Input: part model. Units: mm. Frame: model coordinates. A direction names the side the tool comes from. Coordinates: 2 decimals unless noted, no trailing zeros. Loops run counter-clockwise (first coordinate to the right, second up) from the corner with the lowest first, then second, coordinate; pieces in that order, holes last. Notation, with made-up numbers: (31.25, -26) - (68.25, -26) arc R21 ccw to (68.25, -2) - close; hole circle Ø2 at (72, 69). An arc over 180 degrees is marked (long way). Use a Markdown table: item, result. Add a question column.
1. Section query C-C on x = -8.75. Return the cut outline in (y, z).
2. Access query for faces 1 (the face through (-13.3, -6, 0)), 2 (the face through (-4.01, -5.69, 39.33)), 3 (the face through (-8.3, -6, -1)), 4 (the face through (-5, -6, 25)). Directions: +Z, -Z, +X, -X, +Y, -Y. A direction counts if a zero-diameter tool reaches every point of the face in a straight line with its end or side. Return the directions, or none.
3. Section query B-B on y = -6. Return the cut outline in (x, z), then the cut area to 3 significant figures.
4. Contact query for flat-ended pins moving along their axis: P1, Ø1.4, axis at y = -7, z = 37, coming from the -X side; P2, Ø4, axis at x = -11, y = -8.5, coming from the +Z side; P3, Ø6.5, axis at x = -2.5, y = -4, coming from the -Z side. Output: stop coordinate, or through.
5. Draft query along Z for faces 5 (the face through (-10.84, -6.62, -2.5)), 6 (the face through (-4, -5.2, 37)), 7 (the face through (-9, -6, 5)), 8 (the face through (-4, -6, 0)). Return one class per face: released by +Z, released by -Z, zero draft, split by the parting line, or undercut.
6. Ray query, L1, parallel to Z at x = -3.5, y = -6; L2, parallel to X at y = -3.75, z = 29; L3, parallel to Z at x = -2.25, y = -1.25. Return the intervals inside material, ascending. Write a range as [from, to].
7. Section query A-A on z = -2.7. Return the cut outline in (x, y).
8. Section query D-D on y = -1.75. Return the cut outline in (x, z).
```python
from build123d import *

# Parameters (mm, degrees)
F1_DEPTH = 12
F2_R     = 0.65
F3_DEPTH = 5
F4_R     = 2.35
F4_R_2   = 0.8
F5_DEPTH = 2


with BuildPart() as f1:
    # F0 (on Front) → F1 (new body)
    with BuildSketch(Plane.XZ):
        Polygon((-13.3, 5), (-13.3, -5), (-8.3, -5), (-8.3, 0), (0, 0), (0, 45), (-5, 45), (-5, 5), align=None)
    extrude(amount=F1_DEPTH)

    # F2 (on face) → F3 (cut)
    with BuildSketch(Plane(origin=(-13.3, 0, 0), x_dir=(0, -1, 0), z_dir=(-1, 0, 0))):
        with Locations((6, -2.7)):
            Circle(F2_R)
    extrude(amount=-F3_DEPTH, mode=Mode.SUBTRACT)

    # F4 (on face) → F5 (cut)
    with BuildSketch(Plane(origin=(-5, 0, 0), x_dir=(0, -1, 0), z_dir=(-1, 0, 0))):
        with Locations((6, 37)):
            Circle(F4_R)
        with Locations((6, 37)):
            Circle(F4_R_2, mode=Mode.SUBTRACT)
    extrude(amount=-F5_DEPTH, mode=Mode.SUBTRACT)


solid = f1.part
```
Resolved:
| question | item | result |
|---|---|---|
| 1 | outline | (-12, -5) - (0, -5) - (0, 5) - (-12, 5) - close; hole circle Ø1.3 at (-6, -2.7) |
| 2 | face 1 | +Z, -Z, -X, +Y, -Y |
| 2 | face 2 | -X |
| 2 | face 3 | -Z, +X, +Y, -Y |
| 2 | face 4 | +Z, -X, +Y, -Y |
| 3 | outline | (-13.3, -5) - (-8.3, -5) - (-8.3, -3.35) - (-13.3, -3.35) - close; (-13.3, -2.05) - (-8.3, -2.05) - (-8.3, 0) - (0, 0) - (0, 45) - (-5, 45) - (-5, 39.35) - (-3, 39.35) - (-3, 37.8) - (-5, 37.8) - (-5, 36.2) - (-3, 36.2) - (-3, 34.65) - (-5, 34.65) - (-5, 5) - (-13.3, 5) - close |
| 3 | area | 279 mm² |
| 4 | P1 | x = -5 |
| 4 | P2 | z = 5 |
| 4 | P3 | z = 0 |
| 5 | face 5 | undercut |
| 5 | face 6 | undercut |
| 5 | face 7 | released by +Z |
| 5 | face 8 | released by -Z |
| 6 | L1 | [0, 34.65], [36.2, 37.8], [39.35, 45] |
| 6 | L2 | [-5, 0] |
| 6 | L3 | [0, 45] |
| 7 | outline | (-13.3, -12) - (-8.3, -12) - (-8.3, -6.65) - (-13.3, -6.65) - close; (-13.3, -5.35) - (-8.3, -5.35) - (-8.3, 0) - (-13.3, 0) - close |
| 8 | outline | (-13.3, -5) - (-8.3, -5) - (-8.3, 0) - (0, 0) - (0, 45) - (-5, 45) - (-5, 5) - (-13.3, 5) - close |
